Job drawing, mm, ordinate dimensions from the low corner. One solid piece. A direction names the side the tool comes from. Coordinates: 2 decimals unless noted, no trailing zeros. Write each loop counter-clockwise with the first axis right and the second up, starting at its lowest first coordinate (ties: lowest second). Pieces come first, ordered by that corner, then holes.
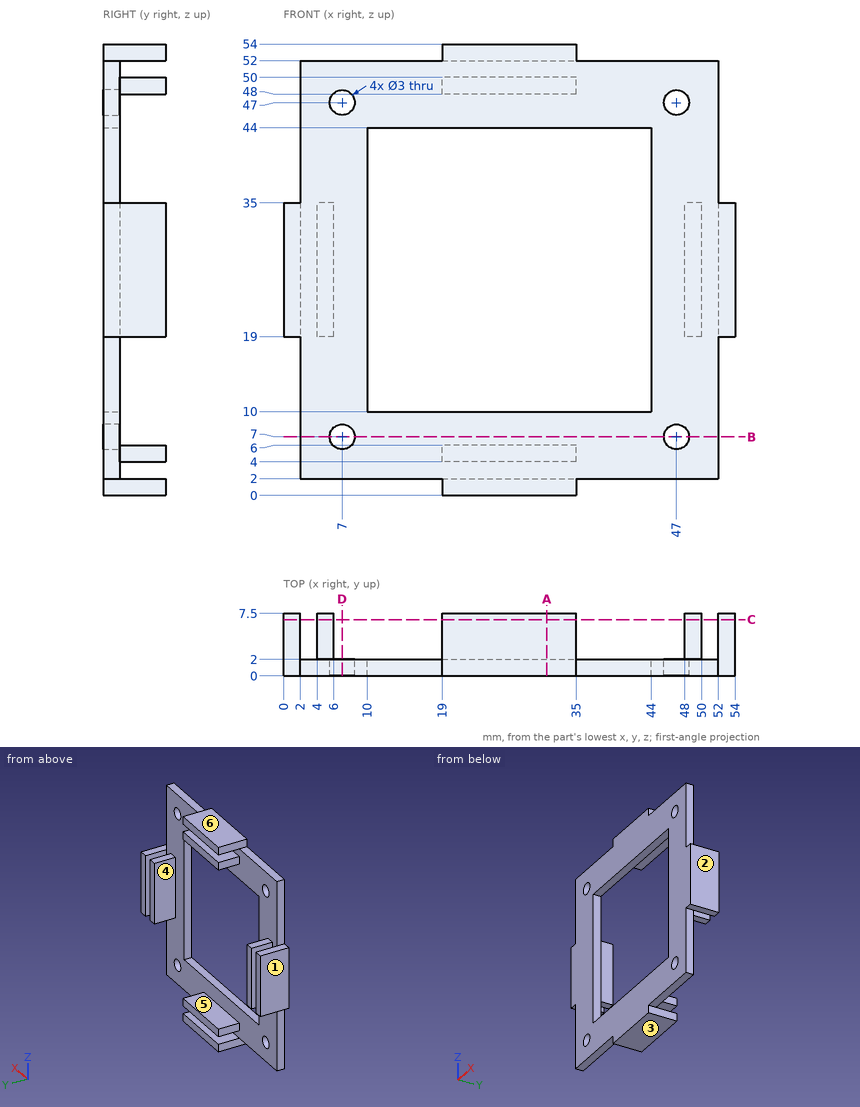
1. Saw through at A-A on x = 31.5. List the corners of the cut face in (y, z), plus the area to 3 significant figures.
Computed values:
outline: (0, 0) - (7.5, 0) - (7.5, 2) - (2, 2) - (2, 4) - (7.5, 4) - (7.5, 6) - (2, 6) - (2, 10) - (0, 10) - close; (0, 44) - (2, 44) - (2, 48) - (7.5, 48) - (7.5, 50) - (2, 50) - (2, 52) - (7.5, 52) - (7.5, 54) - (0, 54) - close
area: 84.0 mm2
2. Flat gauge pins, fed straight in: pin 1 (1.5 mm diameter, centred on x = 14, y = 3, fed in from +Z); pin 2 (1 mm diameter, centred on y = 5.5, z = 49.5, fed in from +X); pin 3 (2 mm diameter, centred on x = 12.5, y = 1, fed in from -Z); pin 4 (1.6 mm diameter, centred on x = 53, y = 4.5, fed in from -Z). Where does each tip first touch, or does it go through?
Computed values:
pin 1: passes through
pin 2: stops at x = 35
pin 3: stops at z = 2
pin 4: stops at z = 19
3. Mould opens along X. For the marked faces 1, 2, 3 and 4 say: +X half, -X half, draft (parallel to the pull), parting line (faces both ways), or undercut.
Computed values:
face 1: -X half
face 2: +X half
face 3: draft
face 4: undercut
4. Probe line 1 along X through (y, z) = (4.25, 27.5); line 2 along X through (y, z) = (1.45, 7). List the from-to ranges inside material, lowest first.
Computed values:
line 1: x = 0 to 2, 4 to 6, 48 to 50, 52 to 54
line 2: x = 2 to 5.5, 8.5 to 45.5, 48.5 to 52
5. Saw through at B-B on z = 7. List the corners of the cut face in (x, y), plus the area to 3 significant figures.
Computed values:
outline: (2, 0) - (5.5, 0) - (5.5, 2) - (2, 2) - close; (8.5, 0) - (45.5, 0) - (45.5, 2) - (8.5, 2) - close; (48.5, 0) - (52, 0) - (52, 2) - (48.5, 2) - close
area: 88.0 mm2
6. Saw through at C-C on y = 6.75. State how many separate pieces and enclosed holes the cut face has, plus the area to 3 significant figures.
Computed values:
separate pieces: 8
enclosed holes: 0
area: 256 mm2
7. 3-axis set-ups, long thin cutter, end or side, ignore diameter. For the marked faces 5 and 6: which of +Z, -Z, +X, -X, +Y, -Y reach the whole face in a straight line?
Computed values:
face 5: +X, -X, +Y
face 6: +Z, +X, -X, +Y, -Y
8. Saw through at D-D on x = 7. List the corners of the cut face in (y, z).
Computed values:
outline: (0, 2) - (2, 2) - (2, 5.5) - (0, 5.5) - close; (0, 8.5) - (2, 8.5) - (2, 45.5) - (0, 45.5) - close; (0, 48.5) - (2, 48.5) - (2, 52) - (0, 52) - close
